Can you work these out from the model? Positions are in its coordinate system, mm. A direction names the side the tool comes from. Coordinates: 2 decimals unless noted, no trailing zeros. Write each loop counter-clockwise with the first axis right and the second up, starting at its lowest first coordinate (ties: lowest second). Pieces come first, ordered by that corner, then holes. Notation, with made-up numbers: M -12,89.5 L 18,89.5 A27 cw 18,122.5 Z; hole C 79.5,-16 d4. An arc over 180 degrees is marked long. Answer as a JSON object with one key per item and string values. Group by question number.
from build123d import *

# Parameters (mm, degrees)
BOSS_EXTRUDE1_DEPTH     = 127
CUT_EXTRUDE1_DEPTH      = 440.390634857
CUT_EXTRUDE1_DEPTH_BACK = 20.32
SKETCH2_W               = 101.6
SKETCH2_H               = 50.8


with BuildPart() as part:
    # Sketch1 → Boss-Extrude1 (new body)
    with BuildSketch(Plane.XY):
        with BuildLine():
            Line((-25.4, -25.4), (-25.4, 228.6))
            ThreePointArc((-25.4, 228.6), (88.9, 342.9), (203.2, 228.6))
            Line((203.2, 228.6), (203.2, -25.4))
            Line((203.2, -25.4), (-25.4, -25.4))
        make_face()
        with BuildLine():
            Line((0, 0), (177.8, 0))
            Line((177.8, 0), (177.8, 228.6))
            ThreePointArc((177.8, 228.6), (88.9, 317.5), (0, 228.6))
            Line((0, 228.6), (0, 0))
        make_face(mode=Mode.SUBTRACT)
    extrude(amount=BOSS_EXTRUDE1_DEPTH)

    # Sketch2 → Cut-Extrude1 (cut, two sides: drawn at the far end of the back side and taken through both)
    with BuildSketch(Plane(origin=(0, 342.9, 0), x_dir=(1, 0, 0), z_dir=(0, 1, 0)).offset(-CUT_EXTRUDE1_DEPTH_BACK)):
        with Locations((88.9, -63.5)):
            Rectangle(SKETCH2_W, SKETCH2_H)
    extrude(amount=CUT_EXTRUDE1_DEPTH + CUT_EXTRUDE1_DEPTH_BACK, mode=Mode.SUBTRACT)


solid = part.part
Q1. On a 3-axis mill with a long thin cutter (end or side, diameter ignored), from which of +Z, -Z, +X, -X, +Y, -Y can I reach the whole of each face in a straight line? I mean faces 5 (the cylindrical face through (90.85, 317.48, 62.61)), 6 (the flat face through (139.7, 327, 64)), 7 (the flat face through (-25.4, 100, 63)). Say none if no direction works.
Q2. If we section it at D-D on z = 105: List the corners of the cut face in (x, y) for me.
Q3. If we section it at B-B on y = 144: List the corners of the cut face in (x, z) for me, and give its area (3 significant figures).
Q4. If we section it at C-C on x = 88.9: List the corners of the cut face in (y, z) for me, and give its area (3 significant figures).
Q5. We'd pull the mould along Z, two halves only. Please class faces 1 (the flat face through (183, 132, 0)), 2 (the flat face through (88, 0, 63)), 3 (the flat face through (38.1, 327, 64)), 4 (the flat face through (88, 330, 88.9)): pulls with the +Z half, pulls with the -Z half, needs draft (parallel to the pull), parting line crosses it, or undercut.
Q6. Will these pins go through, and if not, where does the flat tip stop? pin 1 (6 mm diameter, centred on x = 111.5, z = 15, fed in from +Y); pin 2 (9.5 mm diameter, centred on y = 328, z = 68.5, fed in from +X); pin 3 (10 mm diameter, centred on x = 79.5, y = 330, fed in from -Z); pin 4 (4 mm diameter, centred on y = 326.5, z = 51.5, fed in from -X).
Q7. If we section it at A-A on z = 52: List the corners of the cut face in (x, y) for me, and give its area (3 significant figures).
Q8. Please list where these lines run through material, in increasing order: L1, parallel to X at y = 98, z = 79; L2, parallel to Y at x = 27.5, z = 31; L3, parallel to Y at x = 66.5, z = 14.
Reply:
{
 "1": {"face 5": "+Z, -Z", "face 6": "+Y", "face 7": "+Z, -Z, -X, +Y, -Y"},
 "2": {"outline": "M -25.4,-25.4 L 203.2,-25.4 L 203.2,228.6 A114.3 ccw -25.4,228.6 Z; hole M 0,0 L 177.8,0 L 177.8,228.6 A88.9 ccw 0,228.6 Z"},
 "3": {"outline": "M -25.4,0 L 0,0 L 0,127 L -25.4,127 Z; M 177.8,0 L 203.2,0 L 203.2,127 L 177.8,127 Z", "area": "6,450 mm^2"},
 "4": {"outline": "M -25.4,0 L 0,0 L 0,127 L -25.4,127 Z; M 317.5,0 L 342.9,0 L 342.9,38.1 L 322.58,38.1 L 322.58,88.9 L 342.9,88.9 L 342.9,127 L 317.5,127 Z", "area": "5,420 mm^2"},
 "5": {"face 1": "pulls with the -Z half", "face 2": "needs draft", "face 3": "undercut", "face 4": "undercut"},
 "6": {"pin 1": "y = 341.21", "pin 2": "x = 152.98", "pin 3": "z = 0", "pin 4": "x = 26.71"},
 "7": {"outline": "M -25.4,-25.4 L 203.2,-25.4 L 203.2,228.6 A114.3 ccw 139.7,330.99 L 139.7,322.58 L 38.1,322.58 L 38.1,330.99 A114.3 ccw -25.4,228.6 Z; hole M 0,0 L 177.8,0 L 177.8,228.6 A88.9 ccw 0,228.6 Z", "area": "23,900 mm^2"},
 "8": {"L1": "-25.4 to 0, 177.8 to 203.2", "L2": "-25.4 to 0, 292.89 to 325.01", "L3": "-25.4 to 0, 314.63 to 340.68"}
}
